```python
from build123d import *

# Parameters (mm, degrees)
SKETCH_1_R                   = 22.5
SKETCH_1_R_2                 = 5
EXTRUDE_1_DEPTH              = 11.5
SKETCH_2_R                   = 1.5
CUT_EXTRUDE_1_DEPTH          = 5.5
CHAMFER_1_SIZE               = 0.5
SKETCH_3_OUTSIDE_W           = 59.934
SKETCH_3_OUTSIDE_H           = 59.934
SKETCH_3_OUTSIDE_W_2         = 38
SKETCH_3_OUTSIDE_H_2         = 38
CUT_EXTRUDE_2_DEPTH          = 9
HOLE_WIZARD_M4_1_D           = 3.3
HOLE_WIZARD_M4_1_DEPTH       = 3
HOLE_WIZARD_M4_1_CSINK_D     = 4.05
HOLE_WIZARD_M4_1_CSINK_ANGLE = 90
HOLE_WIZARD_M4_1_TIP         = 0.991420021


with BuildPart() as part:
    # 草图1 → 凸台-拉伸1 (new body)
    with BuildSketch(Plane.XY):
        Circle(SKETCH_1_R)
        Circle(SKETCH_1_R_2, mode=Mode.SUBTRACT)
    extrude(amount=EXTRUDE_1_DEPTH)

    # 草图2 → 切除-拉伸1 (cut)
    with BuildSketch(Plane.XY.offset(11.5)):
        with Locations((0, 17)):
            Circle(SKETCH_2_R)
        with Locations((17, 0)):
            Circle(SKETCH_2_R)
        with Locations((0, -17)):
            Circle(SKETCH_2_R)
        with Locations((-17, 0)):
            Circle(SKETCH_2_R)
    extrude(amount=-CUT_EXTRUDE_1_DEPTH, mode=Mode.SUBTRACT)

    # 倒角1
    chamfer_1_edges = [part.edges().sort_by_distance(p)[0] for p in [
        (-22.5, 0, 11.5),
    ]]
    chamfer(chamfer_1_edges, length=CHAMFER_1_SIZE)

    # 草图3 outside → 切除-拉伸2 (cut)
    with BuildSketch(Plane(origin=(0, 0, 0), x_dir=(-1, 0, 0), z_dir=(0, 0, -1))):
        Rectangle(SKETCH_3_OUTSIDE_W, SKETCH_3_OUTSIDE_H)
        Rectangle(SKETCH_3_OUTSIDE_W_2, SKETCH_3_OUTSIDE_H_2, mode=Mode.SUBTRACT)
    extrude(amount=-CUT_EXTRUDE_2_DEPTH, mode=Mode.SUBTRACT)

    # M4 螺纹孔1
    with Locations(Plane(origin=(0, 0, 0), x_dir=(-1, 0, 0), z_dir=(0, 0, -1))):
        with Locations((0, -15.5), (0, 15.5)):
            CounterSinkHole(HOLE_WIZARD_M4_1_D / 2, HOLE_WIZARD_M4_1_CSINK_D / 2, depth=HOLE_WIZARD_M4_1_DEPTH, counter_sink_angle=HOLE_WIZARD_M4_1_CSINK_ANGLE)
            with Locations((0, 0, -(HOLE_WIZARD_M4_1_DEPTH + HOLE_WIZARD_M4_1_TIP / 2))):  # 118° drill point
                Cone(0, HOLE_WIZARD_M4_1_D / 2, HOLE_WIZARD_M4_1_TIP, mode=Mode.SUBTRACT)


solid = part.part
```
Geometry check sheet. Reference: the model listing, model coordinates, mm. A direction names the side the tool comes from. Coordinates: 2 decimals unless noted, no trailing zeros. Order: outer loops, then holes, each group sorted by start corner. A loop starts at its lowest first (then second) coordinate and runs counter-clockwise, first axis right, second up. Notation, with made-up numbers: (86, -4.5) - (121, -4.5) arc R16 cw to (121, 15.5) - close; hole circle Ø6 at (43.5, 58.25). An arc over 180 degrees is marked (long way). Answer in a Markdown table with one row per item. Add a question column.
1. Section check A-A (y = 0). Enter the section's corners in (x, z), plus the area to 3 significant figures.
2. Gauge pin test, flat ends, axial feed: pin 1 Ø3 at (x, y) = (1, -21) entering from -Z; pin 2 Ø2.5 at (y, z) = (-3.5, 5.5) entering from -X; pin 3 Ø4.5 at (x, z) = (0, 6.5) entering from -Y. Record the tip position at first contact, or that the pin passes through.
3. Material ranges on L1, parallel to Y at x = 0, z = 6.25; L2, parallel to Y at x = 0, z = 1.75; L3, parallel to Z at x = -16.5, y = -0.5, recorded low to high. Write a range as [from, to].
4. Access from +Z, -Z, +X, -X, +Y, -Y to the whole of each face (thin tool, end or side, straight path). Record for faces 1 (the face through (0, 20, 9)), 2 (the face through (-4, 4, 0)), 3 (the face through (-0.195, 18.487, 8.788)), 4 (the face through (-0.4, 13.9, 1.7)).
5. Draft check along X on faces 5 (the face through (0, -17, 6)), 6 (the face through (-18.5, 0.07, 8.79)), 7 (the face through (0, -19, 4)), 8 (the face through (19, 0, 4)). Enter one of: +X half, -X half, draft (parallel to the pull), parting line (faces both ways), or undercut.
6. Section check B-B (z = 7). Enter the section's corners in (x, y).
Data:
| question | item | result |
|---|---|---|
| 1 | outline | (-22.5, 9) - (-19, 9) - (-19, 0) - (-5, 0) - (-5, 11.5) - (-15.5, 11.5) - (-15.5, 6) - (-18.5, 6) - (-18.5, 11.5) - (-22, 11.5) - (-22.5, 11) - close; (5, 0) - (19, 0) - (19, 9) - (22.5, 9) - (22.5, 11) - (22, 11.5) - (18.5, 11.5) - (18.5, 6) - (15.5, 6) - (15.5, 11.5) - (5, 11.5) - close |
| 1 | area | 306 mm² |
| 2 | pin 1 | stops at z = 9 |
| 2 | pin 2 | stops at x = -19 |
| 2 | pin 3 | stops at y = -19 |
| 3 | L1 | y = [-19, -18.5], [-15.5, -5], [5, 15.5], [18.5, 19] |
| 3 | L2 | y = [-19, -17.15], [-13.85, -5], [5, 13.85], [17.15, 19] |
| 3 | L3 | z = [0, 6] |
| 4 | face 1 | -Z, +X, -X, +Y |
| 4 | face 2 | -Z, +X, -X, +Y, -Y |
| 4 | face 3 | +Z |
| 4 | face 4 | -Z |
| 5 | face 5 | undercut |
| 5 | face 6 | undercut |
| 5 | face 7 | draft |
| 5 | face 8 | +X half |
| 6 | outline | (-19, -12.05) arc R22.5 ccw to (-12.05, -19) - (12.05, -19) arc R22.5 ccw to (19, -12.05) - (19, 12.05) arc R22.5 ccw to (12.05, 19) - (-12.05, 19) arc R22.5 ccw to (-19, 12.05) - close; hole circle Ø3 at (-17, 0); hole circle Ø10 at (0, 0); hole circle Ø3 at (0, -17); hole circle Ø3 at (0, 17); hole circle Ø3 at (17, 0) |
